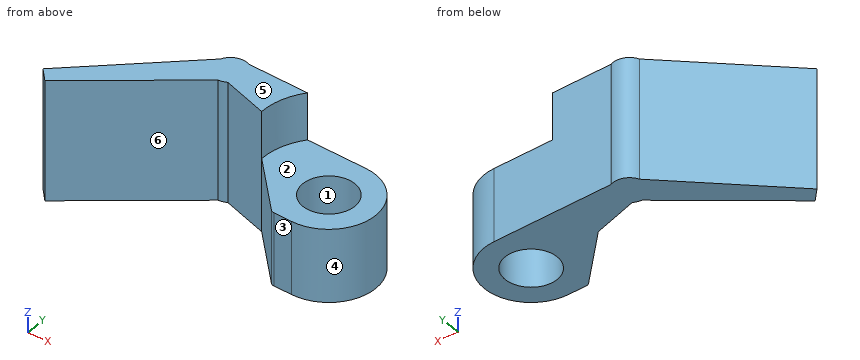
```python
from build123d import *

# Parameters (mm, degrees)
BOSS_EXTRUDE1_DEPTH = 23
SKETCH4_R           = 5
CUT_EXTRUDE3_DEPTH  = 28
CUT_EXTRUDE6_START  = -9
CUT_EXTRUDE6_DEPTH  = 9


with BuildPart() as part:
    # Sketch1 → Boss-Extrude1 (new body)
    with BuildSketch(Plane.XY):
        with BuildLine():
            Line((-26.278110913, -11.347842937), (-28.372166089, -9.043842083))
            Line((-28.372166089, -9.043842083), (-7.990208081, 9.462215656))
            ThreePointArc((-7.990208081, 9.462215656), (-6.229501786, 11.136017118), (-3.800938061, 11.07456612))
            Line((-3.800938061, 11.07456612), (-3.637536714, 11.001987755))
            Line((-3.637536714, 11.001987755), (19.793985679, 9.88969345))
            ThreePointArc((19.793985679, 9.88969345), (28.356197765, 0.474073738), (18.940578052, -8.088138348))
            Line((18.940578052, -8.088138348), (15.348738563, -7.91649311))
            ThreePointArc((15.348738563, -7.91649311), (14.978028358, -7.825889172), (14.668239185, -7.603030926))
            Line((14.668239185, -7.603030926), (5.35012395, 2.296550983))
            Line((5.35012395, 2.296550983), (-3.419163159, 5.255947346))
            ThreePointArc((-3.419163159, 5.255947346), (-4.191805611, 4.94513719), (-5.014133862, 4.813396687))
            Line((-5.014133862, 4.813396687), (-26.278110913, -11.347842937))
        make_face()
    extrude(amount=BOSS_EXTRUDE1_DEPTH)

    # Sketch4 → Cut-Extrude3 (cut)
    with BuildSketch(Plane(origin=(0, 0, 0), x_dir=(-1, 0, 0), z_dir=(0, 0, -1))):
        with Locations((-19.367281866, 0.900777551)):
            Circle(SKETCH4_R)
    extrude(amount=-CUT_EXTRUDE3_DEPTH, mode=Mode.SUBTRACT)

    # Sketch5 → Cut-Extrude6 (cut)
    with BuildSketch(Plane.XY.offset(23).offset(CUT_EXTRUDE6_START)):
        with BuildLine():
            Line((8.078224483, 10.445840603), (19.793985679, 9.88969345))
            ThreePointArc((19.793985679, 9.88969345), (28.356197765, 0.474073738), (18.940578052, -8.088138348))
            Line((18.940578052, -8.088138348), (15.348738563, -7.91649311))
            ThreePointArc((15.348738563, -7.91649311), (14.978028358, -7.825889172), (14.668239185, -7.603030926))
            Line((14.668239185, -7.603030926), (5.35012395, 2.296550983))
            ThreePointArc((5.35012395, 2.296550983), (5.975547098, 6.618462626), (8.078224483, 10.445840603))
        make_face()
    extrude(amount=CUT_EXTRUDE6_DEPTH, mode=Mode.SUBTRACT)


solid = part.part
```
Verification items for the finished model (mm, model axes). Face numbers are marked on the shaded views. A direction names the side the tool comes from. Round coordinates to 2 decimals unless told otherwise and drop trailing zeros. Write each loop counter-clockwise with the first axis right and the second up, starting at its lowest first coordinate (ties: lowest second). Pieces come first, ordered by that corner, then holes.
1. Gauge pin test, flat ends, axial feed: P1, Ø8, axis at x = 19.37, y = 0.9, coming from the +Z side; P2, Ø1, axis at x = 20.5, z = 11.5, coming from the +Y side; P3, Ø2, axis at y = 7, z = 8.5, coming from the +X side; P4, Ø1, axis at y = -5.5, z = 6, coming from the -X side. Record the tip position at first contact, or that the pin passes through.
2. Section check D-D on y = -2.25. Enter the section's corners in (x, z).
3. Access from +Z, -Z, +X, -X, +Y, -Y to the whole of each face (thin tool, end or side, straight path). Record for the marked faces 5 and 6.
4. Scan lines: L1, parallel to X at y = -1.5, z = 4.25; L2, parallel to X at y = -2.25, z = 2.25; L3, parallel to Z at x = 22, y = 9.25. Record each from-to range of solid material in increasing order.
5. Section check C-C on z = 17. Enter the section's corners in (x, y), plus the area to 3 significant figures.
6. Section check A-A on y = -5.75. Enter the section's corners in (x, z), plus the area to 3 significant figures.
7. Section check B-B on x = 16. Enter the section's corners in (y, z).
8. Draft check along Y on the marked faces 1, 2, 3 and 4. Enter one of: +Y half, -Y half, draft (parallel to the pull), parting line (faces both ways), or undercut.
Answer:
1. P1: passes through
1. P2: stops at y = 9.88
1. P3: stops at x = 26.78
1. P4: stops at x = -25.02
2. outline: (-20.89, 0) - (-14.31, 0) - (-14.31, 23) - (-20.89, 23) - close; (9.63, 0) - (15.48, 0) - (15.48, 14) - (9.63, 14) - close; (23.25, 0) - (27.8, 0) - (27.8, 14) - (23.25, 14) - close
3. face 5: +Z, +X, -X, +Y, -Y
3. face 6: +Z, -Z, -Y
4. L1: x = -20.06 to -13.32, 8.92 to 14.98, 23.75 to 28.04
4. L2: x = -20.89 to -14.31, 9.63 to 15.48, 23.25 to 27.8
4. L3: z = 0 to 14
5. outline: (-28.37, -9.04) - (-26.28, -11.35) - (-5.01, 4.81) arc R3.73 ccw to (-3.42, 5.26) - (5.35, 2.3) arc R12.24 cw to (8.08, 10.45) - (-3.64, 11) - (-3.8, 11.07) arc R3.17 ccw to (-7.99, 9.46) - close
5. area: 206 mm2
6. outline: (-24.74, 0) - (-18.91, 0) - (-18.91, 23) - (-24.74, 23) - close; (12.92, 0) - (25.43, 0) - (25.43, 14) - (12.92, 14) - close
6. area: 309 mm2
7. outline: (-7.95, 0) - (-2.8, 0) - (-2.8, 14) - (-7.95, 14) - close; (4.6, 0) - (10.07, 0) - (10.07, 14) - (4.6, 14) - close
8. face 1: undercut
8. face 2: draft
8. face 3: -Y half
8. face 4: parting line
